from build123d import *

# Parameters (mm, degrees)
F0_W      = 317.5
F0_H      = 215.9
F1_DEPTH  = 6.35
F2_W      = 317.5
F2_H      = 292.1
F3_DEPTH  = 6.35
F4_W      = 215.9
F4_H      = 292.1
F5_DEPTH  = 6.35
F7_W      = 215.9
F7_H      = 292.1
F8_DEPTH  = 6.35
F10_W     = 317.5
F10_H     = 317.5
F11_DEPTH = 6.35
F14_W     = 317.5
F14_H     = 228.6
F15_DEPTH = 6.35
F16_W     = 101.6
F16_H     = 38.1
F17_DEPTH = 6.35
F18_W     = 101.6
F18_H     = 38.1
F19_DEPTH = 6.35
F20_W     = 317.5
F20_H     = 38.1
F21_DEPTH = 6.35


with BuildPart() as f1:
    # F0 (on Top) → F1 (new body)
    with BuildSketch(Plane.XY):
        with Locations((158.75, -107.95)):
            Rectangle(F0_W, F0_H)
    extrude(amount=-F1_DEPTH)

    # F2 (on Front) → F3 (join)
    with BuildSketch(Plane.XZ):
        with Locations((158.75, 146.05)):
            Rectangle(F2_W, F2_H)
    extrude(amount=F3_DEPTH)

    # F4 (on Right) → F5 (join)
    with BuildSketch(Plane.YZ):
        with Locations((-107.95, 146.05)):
            Rectangle(F4_W, F4_H)
    extrude(amount=F5_DEPTH)

    # F7 (on offset) → F8 (join)
    with BuildSketch(Plane.YZ.offset(317.5)):
        with Locations((-107.95, 146.05)):
            Rectangle(F7_W, F7_H)
    extrude(amount=-F8_DEPTH)

    # F10 (on offset) → F11 (join)
    with BuildSketch(Plane.XY.offset(292.1)):
        with Locations((158.75, -158.75)):
            Rectangle(F10_W, F10_H)
    extrude(amount=F11_DEPTH)

    # F14 (on offset) → F15 (join)
    with BuildSketch(Plane.XZ.offset(215.9)):
        with Locations((158.75, 114.3)):
            Rectangle(F14_W, F14_H)
    extrude(amount=-F15_DEPTH)

    # F16 (on face) → F17 (join)
    with BuildSketch(Plane.YZ.offset(317.5)):
        with Locations((-266.7, 279.4)):
            Rectangle(F16_W, F16_H)
    extrude(amount=-F17_DEPTH)

    # F18 (on face) → F19 (join)
    with BuildSketch(Plane(origin=(0, 0, 0), x_dir=(0, -1, 0), z_dir=(-1, 0, 0))):
        with Locations((266.7, 279.4)):
            Rectangle(F18_W, F18_H)
    extrude(amount=-F19_DEPTH)

    # F20 (on offset) → F21 (join)
    with BuildSketch(Plane.XZ.offset(317.5)):
        with Locations((158.75, 279.5041836309)):
            Rectangle(F20_W, F20_H)
    extrude(amount=F21_DEPTH)


solid = f1.part
For this review, take the finished solid that the model builds, in its own axes (mm). A direction names the side the tool comes from. Give positions to 0.01 mm unless a question says otherwise; leave off trailing zeros. Loops run counter-clockwise (first coordinate to the right, second up) from the corner with the lowest first, then second, coordinate; pieces in that order, holes last. Notation, with made-up numbers: M 14,6 L 24,6 A16 ccw 24,15 Z; hole C 7,-10 d6. An arc over 180 degrees is marked long. Put each result on its own line as item: value. Start each with the question number.
(1) Add section B-B, the plane y = -133.5. Write out the cut boundary in (x, z), then the cut area to 3 significant figures.
(2) For pin 1 (12 mm diameter, centred on x = 94, y = -172.5, fed in from +Z); pin 2 (3 mm diameter, centred on x = 4, y = -274.5, fed in from -Z); pin 3 (8 mm diameter, centred on x = 105, z = 61.5, fed in from -Y), all flat-tipped, find the tip position at first contact; note any pin that passes through.
(3) Wall thickness on L1, parallel to X at y = -124, z = 245; L2, parallel to Y at x = 94, z = 152; L3, parallel to Z at x = 47.5, y = -133: over which ranges is each line inside the solid? List them lowest first.
(4) The part is to be moulded in two halves that separate along X. For faces 1 (the flat face through (157, -6.35, 148)), 2 (the flat face through (157, -157, 298.45)), 3 (the flat face through (157, -160, 292.1)), 4 (the flat face through (317.5, -124, 144)), say which applies: +X half, -X half, draft (parallel to the pull), parting line (faces both ways), or undercut.
(5) Add section D-D, the plane z = 242. Write out the cut boundary in (x, y).
(6) Add section A-A, the plane z = 165. Write out the cut boundary in (x, y).
(7) Add section C-C, the plane x = 123.5. Write out the cut boundary in (y, z), then the cut area to 3 significant figures.
(8) Machinability: for faces 5 (the flat face through (161, -215.9, 95)), 6 (the flat face through (311.15, -130, 148)), 7 (the flat face through (157, -317.5, 276)), which of the approach directions +Z, -Z, +X, -X, +Y, -Y give a long, thin tool a straight path to every point of the face, cutting with its end or side? Answer none if there is none.
Result:
1. outline: M 0,-6.35 L 317.5,-6.35 L 317.5,298.45 L 0,298.45 Z; hole M 6.35,0 L 311.15,0 L 311.15,292.1 L 6.35,292.1 Z
1. area: 7,740 mm^2
2. pin 1: stops at z = 298.45
2. pin 2: stops at z = 260.35
2. pin 3: stops at y = -215.9
3. L1: x = 0 to 6.35, 311.15 to 317.5
3. L2: y = -215.9 to -209.55, -6.35 to 0
3. L3: z = -6.35 to 0, 292.1 to 298.45
4. face 1: undercut
4. face 2: draft
4. face 3: undercut
4. face 4: +X half
5. outline: M 0,-215.9 L 6.35,-215.9 L 6.35,-6.35 L 311.15,-6.35 L 311.15,-215.9 L 317.5,-215.9 L 317.5,0 L 0,0 Z
6. outline: M 0,-215.9 L 317.5,-215.9 L 317.5,0 L 0,0 Z; hole M 6.35,-209.55 L 311.15,-209.55 L 311.15,-6.35 L 6.35,-6.35 Z
7. outline: M -323.85,260.45 L -317.5,260.45 L -317.5,292.1 L -6.35,292.1 L -6.35,0 L -209.55,0 L -209.55,228.6 L -215.9,228.6 L -215.9,-6.35 L 0,-6.35 L 0,298.45 L -317.5,298.45 L -317.5,298.55 L -323.85,298.55 Z
7. area: 6,940 mm^2
8. face 5: -Z, +X, -X, -Y
8. face 6: none
8. face 7: -Z
